Geometry check sheet. Reference: the model listing, model coordinates, mm. Face numbers are marked on the shaded views. A direction names the side the tool comes from. Coordinates: 2 decimals unless noted, no trailing zeros. Order: outer loops, then holes, each group sorted by start corner. A loop starts at its lowest first (then second) coordinate and runs counter-clockwise, first axis right, second up. Notation, with made-up numbers: M 19,65.5 L 59,65.5 A18 cw 59,79.5 Z; hole C 7.25,61.5 d11. An arc over 180 degrees is marked long. Use CSV: the item, a comma, the result in double quotes. Start each with the question number.
```python
from build123d import *

# Parameters (mm, degrees)
F0_W     = 68.36
F0_H     = 38.402704
F1_DEPTH = 10
F2_R     = 7.466851
F3_DEPTH = 5
F4_W     = 42.948617
F4_H     = 26.389016
F5_DEPTH = 1
F6_R     = 4.253524
F7_DEPTH = 1


with BuildPart() as f1:
    # F0 (on Top) → F1 (new body)
    with BuildSketch(Plane.XY):
        with Locations((-0.695145, -0.397226)):
            Rectangle(F0_W, F0_H)
    extrude(amount=F1_DEPTH)

    # F2 (on face) → F3 (cut)
    with BuildSketch(Plane.XY.offset(10)):
        Circle(F2_R)
    extrude(amount=-F3_DEPTH, mode=Mode.SUBTRACT)

    # F4 (on face) → F5 (join)
    with BuildSketch(Plane.YZ.offset(33.484855)):
        with Locations((1.87573, 13.194508)):
            Rectangle(F4_W, F4_H)
    extrude(amount=F5_DEPTH)

    # F6 (on face) → F7 (cut)
    with BuildSketch(Plane.YZ.offset(34.484855)):
        with Locations((0, 18.462041)):
            Circle(F6_R)
    extrude(amount=-F7_DEPTH, mode=Mode.SUBTRACT)


solid = f1.part
```
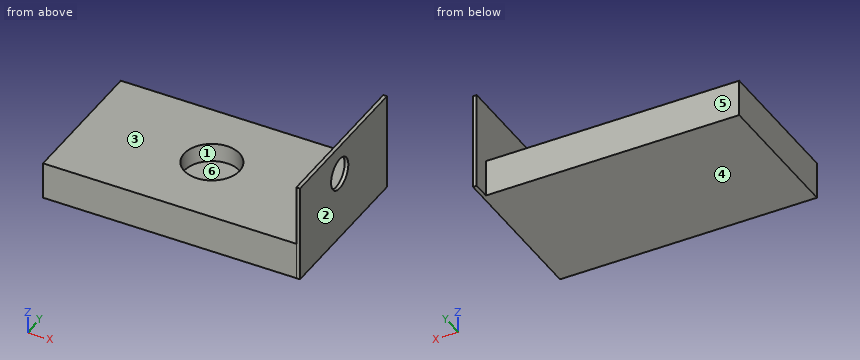
1) Material ranges on line 1 along Y through (x, z) = (0, 8.75); line 2 along Z through (x, y) = (34.2, 0); line 3 along Y through (x, z) = (14, 9), recorded low to high.
2) Set-up check for the marked faces 4, 5 and 6: record each of +Z, -Z, +X, -X, +Y, -Y from which the full face is reachable in a straight line by a thin tool's end or side.
3) Gauge pin test, flat ends, axial feed: P1, Ø13.5, axis at y = 0, z = 18.46, coming from the +X side; P2, Ø19, axis at x = 4.5, y = -5.5, coming from the +Z side; P3, Ø8, axis at x = -27, z = 17, coming from the +Y side; P4, Ø5, axis at x = 16, z = 5.5, coming from the +Y side. Record the tip position at first contact, or that the pin passes through.
4) Section check A-A on y = 0. Record the boundary of the cut face in (x, z), then the cut area to 3 significant figures.
5) Section check D-D on x = 0. Record the boundary of the cut face in (y, z).
6) Section check C-C on z = 20. Record the boundary of the cut face in (x, y), then the cut area to 3 significant figures.
7) Draft check along X on the marked faces 1, 2 and 3. Enter one of: +X half, -X half, draft (parallel to the pull), parting line (faces both ways), or undercut.
8) Section check B-B on z = 9. Record the boundary of the cut face in (x, y).
Results are:
1,line 1,"y = -19.6 to -7.47, 7.47 to 18.8"
1,line 2,"z = 0 to 14.21, 22.72 to 26.39"
1,line 3,"y = -19.6 to 18.8"
2,face 4,"-Z, +X, -X, +Y, -Y"
2,face 5,"+Z, -Z, -X, +Y"
2,face 6,"+Z"
3,P1,"stops at x = 34.48"
3,P2,"stops at z = 10"
3,P3,"passes through"
3,P4,"stops at y = 18.8"
4,outline,"M -34.88,0 L 34.48,0 L 34.48,14.21 L 33.48,14.21 L 33.48,10 L 7.47,10 L 7.47,5 L -7.47,5 L -7.47,10 L -34.88,10 Z; M 33.48,22.72 L 34.48,22.72 L 34.48,26.39 L 33.48,26.39 Z"
4,area,"627 mm²"
5,outline,"M -19.6,0 L 18.8,0 L 18.8,10 L 7.47,10 L 7.47,5 L -7.47,5 L -7.47,10 L -19.6,10 Z"
6,outline,"M 33.48,-19.6 L 34.48,-19.6 L 34.48,-3.97 L 33.48,-3.97 Z; M 33.48,3.97 L 34.48,3.97 L 34.48,23.35 L 33.48,23.35 Z"
6,area,"35.0 mm²"
7,face 1,"undercut"
7,face 2,"+X half"
7,face 3,"draft"
8,outline,"M -34.88,-19.6 L 34.48,-19.6 L 34.48,23.35 L 33.48,23.35 L 33.48,18.8 L -34.88,18.8 Z; hole C 0,0 d14.93"
